Read the model definition and answer for the solid it produces. Units are mm, in the model's axes. A direction names the side the tool comes from. Coordinates: 2 decimals unless noted, no trailing zeros. Loops run counter-clockwise (first coordinate to the right, second up) from the corner with the lowest first, then second, coordinate; pieces in that order, holes last. Notation, with made-up numbers: (51, 68) - (96, 68) arc R28 ccw to (96, 91) - close; hole circle Ø3 at (6.5, 56.5). An arc over 180 degrees is marked (long way). Use one line per item in the form item = value. Start each with the question number.
1) Each of these flat-tipped pins is pushed along its axis until it touches: P1, Ø5, axis at y = 2, z = -37.5, coming from the +X side; P2, Ø2.5, axis at x = -43, y = 4.5, coming from the -Z side; P3, Ø3, axis at y = 5, z = 3.5, coming from the -X side; P4, Ø1, axis at x = 63, z = -37, coming from the +Y side. Where does it stop, or does it pass through?
2) Which of the six approach directions +Z, -Z, +X, -X, +Y, -Y give full straight-line access (tool end or side, diameter ignored) to faces 1 (the face through (-46.5, 4, 24)), 2 (the face through (-44, 4, 26.5)), 3 (the face through (-41.5, 4, 24)), 4 (the face through (-44, 4, 21.5)), 5 (the face through (1, -1.75, 1))?
3) A cutting plane is placed at A-A (z = 18.5). Give the vertices of the cut face in (x, y), and give its area (4 significant figures).
4) A cutting plane is placed at B-B (y = 4.75). Give the vertices of the cut face in (x, z), and give its area (3 significant figures).
5) Consider line 1 (Y direction, x = 15, z = 0); line 2 (Z direction, x = -44.5, y = 6). Determine where each line is inside the solid, lowest interval first.
Autodesk Inventor part; units mm, degrees
ref_plane "YZ Plane" through (0, 0, 0) normal (1, 0, 0) x (0, 1, 0)
ref_plane "XZ Plane" through (0, 0, 0) normal (0, 1, 0) x (-1, 0, 0)
ref_plane "XY Plane" through (0, 0, 0) normal (0, 0, 1) x (1, 0, 0)
sketch "Náčrt1" plane through (0, 0, 0) normal (0, 1, 0) x (-1, 0, 0)
  line L0 (0, -93.1) -> (0, 93.1)
  line L1 (-121.1, 0) -> (121.1, 0)
  line L2 (86.5, 66.5) -> (-86.5, 66.5)
  line L3 (-86.5, 66.5) -> (-86.5, -66.5)
  line L4 (-86.5, -66.5) -> (86.5, -66.5)
  line L5 (86.5, -66.5) -> (86.5, 66.5)
  point P0 (0, 0)
  dimension "d0" = 133
  dimension "d1" = 173
extrude "Vysunutí1" add sketch "Náčrt1" along normal mid plane 3.5
sketch "Náčrt2" plane through (0, 1.75, 0) normal (0, 1, 0) x (1, 0, 0)
  line L0 (-46.5, -26.5) -> (-41.5, -26.5)
  line L1 (-41.5, -26.5) -> (-41.5, -21.5)
  line L2 (-41.5, -21.5) -> (-46.5, -21.5)
  line L3 (-46.5, -21.5) -> (-46.5, -26.5)
  line L4 (-86.5, -66.5) -> (86.5, -66.5)
  line L5 (-86.5, 66.5) -> (-86.5, -66.5)
  point P0 (0, 0)
  dimension "d4" = 5
  dimension "d5" = 5
  dimension "d6" = 40
  dimension "d7" = 40
extrude "Vysunutí2" add sketch "Náčrt2" along normal blind 5
properties part number "Cabinet - left"
Found:
q1.P1 = 86.5
q1.P2 = 21.5
q1.P3 = through
q1.P4 = 1.75
q2.face_1 = +Z, -Z, -X, +Y
q2.face_2 = +Z, +X, -X, +Y
q2.face_3 = +Z, -Z, +X, +Y
q2.face_4 = -Z, +X, -X, +Y
q2.face_5 = +Z, -Z, +X, -X, -Y
q3.outline = (-86.5, -1.75) - (86.5, -1.75) - (86.5, 1.75) - (-86.5, 1.75) - close
q3.area = 605.5 mm^2
q4.outline = (-46.5, 21.5) - (-41.5, 21.5) - (-41.5, 26.5) - (-46.5, 26.5) - close
q4.area = 25.0 mm^2
q5.line_1 = -1.75 to 1.75
q5.line_2 = 21.5 to 26.5
